Work out the finished part from the listing and answer in its coordinate system (mm). Face numbers are marked on the shaded views. A direction names the side the tool comes from. Coordinates: 2 decimals unless noted, no trailing zeros. Write each loop counter-clockwise with the first axis right and the second up, starting at its lowest first coordinate (ties: lowest second). Pieces come first, ordered by that corner, then holes. Notation, with made-up numbers: (-12.5, 16.25) - (23.5, 16.25) arc R31 ccw to (23.5, 40.25) - close; hole circle Ø10 at (28.25, 64). An arc over 180 degrees is marked (long way). Use a Markdown table: item, result. Add a question column.
(1) The part is cut by section C-C, the plane x = -9. Give the vertices of the cut face in (y, z) (1 decimal), then the cut area to 3 significant figures.
(2) A tool of negligible diameter and unlimited length cuts with its end or side. For the marked faces 1, 2 and 3, from which of +Z, -Z, +X, -X, +Y, -Y can it reach the whole face along a straight path? Write none if from no direction.
(3) Given pin 1 Ø1.6 at (x, z) = (-5.5, -0.5) entering from -Y; pin 2 Ø1 at (y, z) = (41, 0.5) entering from +X; pin 3 Ø1.6 at (x, z) = (-2.5, 0.5) entering from +Y; pin 4 Ø1.6 at (y, z) = (55, 0.5) entering from +X (3 decimals), each flat-ended and moving along its own axis, determine where each tip first touches the part or whether it passes through.
(4) Find the intervals of material crossed by line 1 (X direction, y = 12.5, z = -0.1) (1 decimal); line 2 (Y direction, x = -25.5, z = 1.15) (3 decimals); line 3 (Y direction, x = -4.5, z = 0.4), in increasing order. Write a range as from..to.
(5) The part is cut by section A-A, the plane y = 27.5. Give the vertices of the cut face in (x, z) (1 decimal).
(6) The part is cut by section B-B, the plane z = 0.6. State how many separate pieces and enclosed holes the cut face has, then the cut area to 3 significant figures.
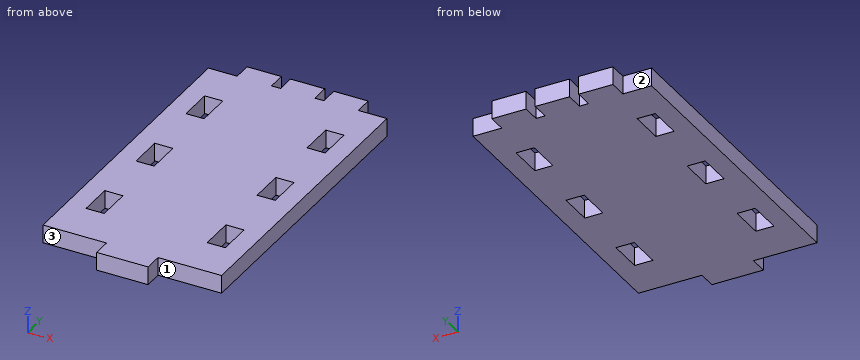
from build123d import *

# Parameters (mm, degrees)
SKETCH1_W           = 3.175
SKETCH1_H           = 6
BOSS_EXTRUDE1_DEPTH = 1.5875


with BuildPart() as part:
    # Sketch1 → Boss-Extrude1 (new body, symmetric)
    with BuildSketch(Plane.XY):
        Polygon((0, 0), (-11.1125, 0), (-11.1125, -3.175), (-20.1125, -3.175), (-20.1125, 0), (-31.225, 0), (-31.225, 53), (-26.2, 53), (-26.2, 56.175), (-20.2, 56.175), (-20.2, 53), (-18.6125, 53), (-18.6125, 56.175), (-12.6125, 56.175), (-12.6125, 53), (-11.025, 53), (-11.025, 56.175), (-5.025, 56.175), (-5.025, 53), (0, 53), align=None)
        with Locations((-5.025, 10.5)):
            Rectangle(SKETCH1_W, SKETCH1_H, mode=Mode.SUBTRACT)
        Polygon((-5.025, 23.5), (-3.4375, 23.5), (-3.4375, 29.5), (-6.6125, 29.5), (-6.6125, 23.5), align=None, mode=Mode.SUBTRACT)
        Polygon((-5.025, 39.5), (-3.4375, 39.5), (-3.4375, 45.5), (-6.6125, 45.5), (-6.6125, 39.5), align=None, mode=Mode.SUBTRACT)
        Polygon((-24.6125, 39.5), (-26.2, 39.5), (-27.7875, 39.5), (-27.7875, 45.5), (-24.6125, 45.5), align=None, mode=Mode.SUBTRACT)
        Polygon((-24.6125, 23.5), (-26.2, 23.5), (-27.7875, 23.5), (-27.7875, 29.5), (-24.6125, 29.5), align=None, mode=Mode.SUBTRACT)
        with Locations((-26.2, 10.5)):
            Rectangle(SKETCH1_W, SKETCH1_H, mode=Mode.SUBTRACT)
    extrude(amount=BOSS_EXTRUDE1_DEPTH, both=True)


solid = part.part
Model answer:
| question | item | result |
|---|---|---|
| 1 | outline | (0, -1.6) - (56.2, -1.6) - (56.2, 1.6) - (0, 1.6) - close |
| 1 | area | 178 mm^2 |
| 2 | face 1 | +Z, -Z, +X, -Y |
| 2 | face 2 | +Z, -Z, -X, +Y |
| 2 | face 3 | +Z, -Z, -X, -Y |
| 3 | pin 1 | y = 0 |
| 3 | pin 2 | x = 0 |
| 3 | pin 3 | y = 53 |
| 3 | pin 4 | x = -5.025 |
| 4 | line 1 | -31.2..-27.8, -24.6..-6.6, -3.4..0 |
| 4 | line 2 | 0..7.5, 13.5..23.5, 29.5..39.5, 45.5..56.175 |
| 4 | line 3 | 0..7.5, 13.5..23.5, 29.5..39.5, 45.5..53 |
| 5 | outline | (-31.2, -1.6) - (-27.8, -1.6) - (-27.8, 1.6) - (-31.2, 1.6) - close; (-24.6, -1.6) - (-6.6, -1.6) - (-6.6, 1.6) - (-24.6, 1.6) - close; (-3.4, -1.6) - (0, -1.6) - (0, 1.6) - (-3.4, 1.6) - close |
| 6 | separate pieces | 1 |
| 6 | enclosed holes | 6 |
| 6 | area | 1,630 mm^2 |
